from build123d import *

# Parameters (mm, degrees)
SKETCH_1_R      = 17.5
EXTRUDE_1_DEPTH = 60
SKETCH_2_R      = 20
EXTRUDE_2_DEPTH = 20
SKETCH_3_R      = 15
EXTRUDE_3_DEPTH = 4
SKETCH_4_R      = 20
EXTRUDE_4_DEPTH = 100
SKETCH_5_R      = 22.5
EXTRUDE_5_DEPTH = 20
SKETCH_6_R      = 15
EXTRUDE_6_DEPTH = 40


with BuildPart() as part:
    # 草图1 → 凸台-拉伸1 (new body)
    with BuildSketch(Plane(origin=(0, 0, 0), x_dir=(1, 0, 0), z_dir=(0, 1, 0))):
        with Locations(Location((0, 0, 0), (0, 0, 270))):
            Circle(SKETCH_1_R)
    extrude(amount=EXTRUDE_1_DEPTH)

    # 草图2 → 凸台-拉伸2 (add)
    with BuildSketch(Plane(origin=(0, 60, 0), x_dir=(1, 0, 0), z_dir=(0, 1, 0))):
        with Locations(Location((0, 0, 0), (0, 0, 270))):
            Circle(SKETCH_2_R)
    extrude(amount=EXTRUDE_2_DEPTH)

    # 草图3 → 凸台-拉伸3 (add)
    with BuildSketch(Plane(origin=(0, 80, 0), x_dir=(1, 0, 0), z_dir=(0, 1, 0))):
        with Locations(Location((0, 0, 0), (0, 0, 270))):
            Circle(SKETCH_3_R)
    extrude(amount=EXTRUDE_3_DEPTH)

    # 草图4 → 凸台-拉伸4 (add)
    with BuildSketch(Plane(origin=(0, 84, 0), x_dir=(1, 0, 0), z_dir=(0, 1, 0))):
        with Locations(Location((0, 0, 0), (0, 0, 270))):
            Circle(SKETCH_4_R)
    extrude(amount=EXTRUDE_4_DEPTH)

    # 草图5 → 凸台-拉伸5 (add)
    with BuildSketch(Plane(origin=(0, 184, 0), x_dir=(1, 0, 0), z_dir=(0, 1, 0))):
        with Locations(Location((0, 0, 0), (0, 0, 270))):
            Circle(SKETCH_5_R)
    extrude(amount=EXTRUDE_5_DEPTH)

    # 草图6 → 凸台-拉伸6 (add)
    with BuildSketch(Plane(origin=(0, 204, 0), x_dir=(1, 0, 0), z_dir=(0, 1, 0))):
        with Locations(Location((0, 0, 0), (0, 0, 270))):
            Circle(SKETCH_6_R)
    extrude(amount=EXTRUDE_6_DEPTH)


solid = part.part
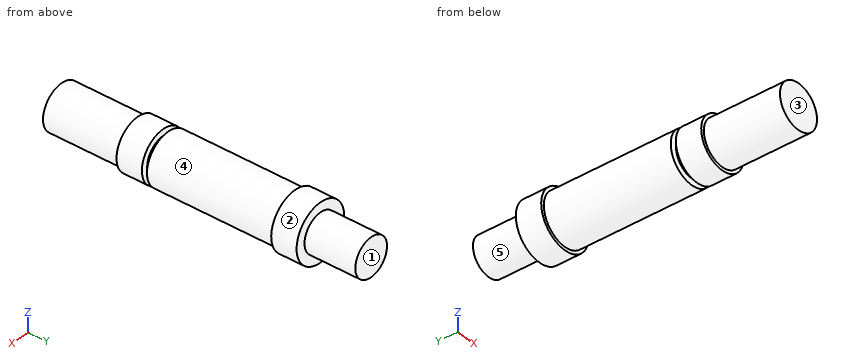
Could you check a few things on this model? Use its own coordinates, in mm. Face numbers are marked on the shaded views. A direction names the side the tool comes from. Give positions to 0.01 mm unless a question says otherwise; leave off trailing zeros. Write each loop counter-clockwise with the first axis right and the second up, starting at its lowest first coordinate (ties: lowest second). Pieces come first, ordered by that corner, then holes. Notation, with made-up numbers: (1.5, 31) - (27.5, 31) arc R17 ccw to (27.5, 50) - close; hole circle Ø1 at (18.5, 44). An arc over 180 degrees is marked (long way). Use CSV: the item, a comma, the result in double quotes. Start each with the question number.
Item 1: If I drill on line 1 along Y through (x, z) = (0.5, 16); line 2 along Y through (x, z) = (-8.5, -17.5); line 3 along X through (y, z) = (149.5, -0.5), over which ranges is the centre line in solid material (lowest first)?
Item 2: I'm going to push flat-ended pins straight in: pin 1 (1 mm diameter, centred on x = -12.5, z = 13, fed in from +Y); pin 2 (12 mm diameter, centred on x = 13, y = 123.5, fed in from +Z) (3 decimals); pin 3 (6 mm diameter, centred on x = -13, z = -9.5, fed in from +Y); pin 4 (10 mm diameter, centred on y = 86.5, z = -10.5, fed in from -X). Where does each tip first touch, or does it pass through?
Item 3: I want a section at C-C, the plane y = 171. Please give me the cut outline in (x, z).
Item 4: I want a section at D-D, the plane y = 210. Please give me the cut outline in (x, z).
Item 5: If we mould it in two halves opening along Z, with no side actions, what happens to the marked faces 1 and 2? For each: pulls with the +Z half, pulls with the -Z half, needs draft (parallel to the pull), parting line crosses it, or undercut.
Item 6: For the marked faces 3, 4 and 5, which set-ups out of +Z, -Z, +X, -X, +Y, -Y let a thin tool reach every point of the face, with its end or its side?
Item 7: I want a section at B-B, the plane z = 0. Please give me the cut outline in (x, y).
Item 8: I want a section at A-A, the plane x = 0. Please give me the cut outline in (y, z), then the cut area to 3 significant figures.
Findings:
1,line 1,"y = 0 to 80, 84 to 204"
1,line 2,"y = 60 to 80, 84 to 204"
1,line 3,"x = -19.99 to 19.99"
2,pin 1,"stops at y = 204"
2,pin 2,"stops at z = 18.735"
2,pin 3,"stops at y = 244"
2,pin 4,"stops at x = -19.23"
3,outline,"circle Ø40 at (0, 0)"
4,outline,"circle Ø30 at (0, 0)"
5,face 1,"needs draft"
5,face 2,"parting line crosses it"
6,face 3,"+Z, -Z, +X, -X, -Y"
6,face 4,"-Y"
6,face 5,"+Y"
7,outline,"(-22.5, 184) - (-20, 184) - (-20, 84) - (-15, 84) - (-15, 80) - (-20, 80) - (-20, 60) - (-17.5, 60) - (-17.5, 0) - (17.5, 0) - (17.5, 60) - (20, 60) - (20, 80) - (15, 80) - (15, 84) - (20, 84) - (20, 184) - (22.5, 184) - (22.5, 204) - (15, 204) - (15, 244) - (-15, 244) - (-15, 204) - (-22.5, 204) - close"
8,outline,"(0, -17.5) - (60, -17.5) - (60, -20) - (80, -20) - (80, -15) - (84, -15) - (84, -20) - (184, -20) - (184, -22.5) - (204, -22.5) - (204, -15) - (244, -15) - (244, 15) - (204, 15) - (204, 22.5) - (184, 22.5) - (184, 20) - (84, 20) - (84, 15) - (80, 15) - (80, 20) - (60, 20) - (60, 17.5) - (0, 17.5) - close"
8,area,"9,120 mm2"
